The listing builds one solid part. Answer for the finished solid, in the listing's coordinates (mm). A direction names the side the tool comes from. Round coordinates to 2 decimals unless told otherwise and drop trailing zeros. Write each loop counter-clockwise with the first axis right and the second up, starting at its lowest first coordinate (ties: lowest second). Pieces come first, ordered by that corner, then holes. Notation, with made-up numbers: (-7.5, 11.25) - (20.5, 11.25) arc R22 ccw to (20.5, 20.25) - close; hole circle Ø2 at (-4.5, 59). An arc over 180 degrees is marked (long way). Use a Markdown table: item, result. Add a question column.
1) A cutting plane is placed at A-A (y = -38.1). Give the vertices of the cut face in (x, z), then the cut area to 3 significant figures.
2) A tool of negligible diameter and unlimited length cuts with its end or side. For faces 1 (the flat face through (-24.774, -82, 36)), 2 (the flat face through (-38, -82, 48.654)), 3 (the cylindrical face through (6.887, -39.753, 48.546)), 4 (the flat face through (-50.174, -82, 36)), 5 (the flat face through (-38, -82, 23.254)), from which of +Z, -Z, +X, -X, +Y, -Y can it reach the whole face along a straight path? Write none if from no direction.
3) A cutting plane is placed at C-C (z = 6). Give the vertices of the cut face in (x, y).
4) Determine the mould class of faces 6 (the flat face through (0.626, -38, 18)), 7 (the cylindrical face through (-34.721, -50.498, 35.421)), 8 (the flat face through (-43, 0, 35)) for opening direction X: +X half, -X half, draft (parallel to the pull), parting line (faces both ways), or undercut.
5) Find the intervals of material crossed by probe 1 along X at (y, z) = (-38, 51); probe 2 along Y at (x, z) = (-67, 4.5); probe 3 along Z at (x, y) = (-27, -78), in increasing order. Write a range as from..to.
6) A cutting plane is placed at B-B (x = -46). Give the vertices of the cut face in (y, z), then the cut area to 3 significant figures.
7) Each of these flat-tipped pins is pushed along its axis until it touches: P1, Ø1.5, axis at x = -57, z = 59.5, coming from the -Y side; P2, Ø4, axis at y = -81, z = 42, coming from the -X side; P3, Ø6.5, axis at y = -82.5, z = 32.5, coming from the +X side; P4, Ø20.5, axis at x = -37.47, y = -38.1, coming from the -Z side. Where does it stop, or does it pass through?
8) A cutting plane is placed at D-D (y = -83). Give the vertices of the cut face in (x, z).
```python
from build123d import *

# Parameters (mm, degrees)
F0_W     = 76.2
F0_H     = 76.2
F1_DEPTH = 76.2
F2_R     = 12.7
F3_DEPTH = 12.7
F5_D     = 25.4
F6_W     = 25.4
F6_H     = 25.4
F7_DEPTH = 12.7
F8_W     = 76.2
F8_H     = 76.2
F9_DEPTH = 12.7


with BuildPart() as f1:
    # F0 (on Front) → F1 (new body)
    with BuildSketch(Plane.XZ):
        with Locations((-37.473612465, 35.9543495976)):
            Rectangle(F0_W, F0_H)
    extrude(amount=F1_DEPTH)

    # F2 (on face) → F3 (join)
    with BuildSketch(Plane.YZ.offset(0.626387535)):
        with Locations((-38.1, 35.9543495976)):
            Circle(F2_R)
    extrude(amount=F3_DEPTH)

    # F5 (through all)
    with Locations(Plane.XY.offset(74.0543495976)):
        with Locations((-37.473612465, -38.1)):
            Hole(F5_D / 2)

    # F6 (on face) → F7 (join)
    with BuildSketch(Plane.XZ.offset(76.2)):
        with Locations((-37.473612465, 35.9543495976)):
            Rectangle(F6_W, F6_H)
    extrude(amount=F7_DEPTH)

    # F8 (on face) → F9 (join)
    with BuildSketch(Plane(origin=(-75.573612465, 0, 0), x_dir=(0, -1, 0), z_dir=(-1, 0, 0))):
        with Locations((38.1, 35.9543495976)):
            Rectangle(F8_W, F8_H)
        Polygon((23.0061305957, 44.0499627439), (48.0005134924, 48.5711156515), (39.4187553165, 24.6647686573), align=None, mode=Mode.SUBTRACT)
        Polygon((39.4187553165, 24.6647686573), (48.0005134924, 48.5711156515), (23.0061305957, 44.0499627439), align=None)
    extrude(amount=F9_DEPTH)


solid = f1.part
```
Entries:
| question | item | result |
|---|---|---|
| 1 | outline | (-88.27, -2.15) - (-50.17, -2.15) - (-50.17, 74.05) - (-88.27, 74.05) - close; (-24.77, -2.15) - (0.63, -2.15) - (0.63, 23.25) - (13.33, 23.25) - (13.33, 48.65) - (0.63, 48.65) - (0.63, 74.05) - (-24.77, 74.05) - close |
| 1 | area | 5,160 mm² |
| 2 | face 1 | +Z, -Z, +X, -Y |
| 2 | face 2 | +Z, +X, -X, -Y |
| 2 | face 3 | +X |
| 2 | face 4 | +Z, -Z, -X, -Y |
| 2 | face 5 | -Z, +X, -X, -Y |
| 3 | outline | (-88.27, -76.2) - (0.63, -76.2) - (0.63, 0) - (-88.27, 0) - close; hole circle Ø25.4 at (-37.47, -38.1) |
| 4 | face 6 | +X half |
| 4 | face 7 | undercut |
| 4 | face 8 | draft |
| 5 | probe 1 | x = -88.27..-50.17, -24.77..0.63 |
| 5 | probe 2 | y = -76.2..0 |
| 5 | probe 3 | z = 23.25..48.65 |
| 6 | outline | (-88.9, 23.25) - (-76.2, 23.25) - (-76.2, -2.15) - (-47.51, -2.15) - (-47.51, 74.05) - (-76.2, 74.05) - (-76.2, 48.65) - (-88.9, 48.65) - close; (-28.69, -2.15) - (0, -2.15) - (0, 74.05) - (-28.69, 74.05) - close |
| 6 | area | 4,690 mm² |
| 7 | P1 | stops at y = -76.2 |
| 7 | P2 | stops at x = -50.17 |
| 7 | P3 | stops at x = -24.77 |
| 7 | P4 | passes through |
| 8 | outline | (-50.17, 23.25) - (-24.77, 23.25) - (-24.77, 48.65) - (-50.17, 48.65) - close |
